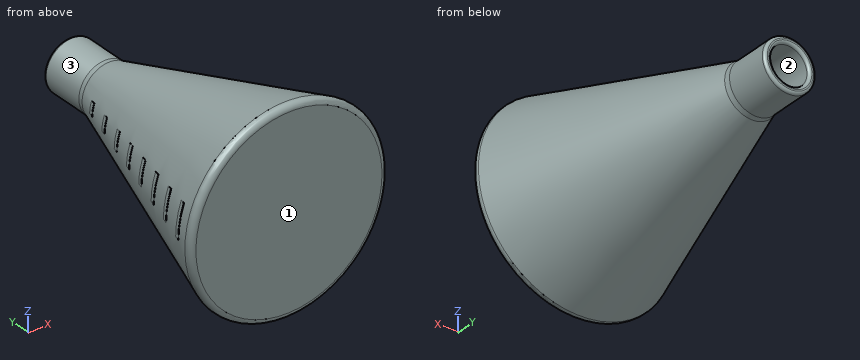
from build123d import *

# Parameters (mm, degrees)
FILLET1_R      = 7.62
FILLET2_R      = 1.27
FILLET3_R      = 2.54
FILLET4_R      = 2.54
REVOLVE2_ANGLE = 20


with BuildPart() as part:
    # Sketch2 → Revolve1 (revolve)
    with BuildSketch(Plane.XY, mode=Mode.PRIVATE) as revolve1_sk:
        Polygon((-11.704475972, 127), (-8.529475972, 127), (-8.529475972, 105.527709861), (-41.475985329, 3.175), (0, 3.175), (0, 0), (-45.672992146, 0), (-11.704475972, 105.527709861), align=None)
    revolve(revolve1_sk.sketch.rotate(Axis((0, 0, 0), (0, 1, 0)), 270), axis=Axis((0, 0, 0), (0, 1, 0)))

    # Fillet1
    fillet1_edges = [part.edges().sort_by_distance(p)[0] for p in [
        (0, 105.527709861, 11.704475972),
    ]]
    fillet(fillet1_edges, radius=FILLET1_R)

    # Fillet2
    fillet2_edges = [part.edges().sort_by_distance(p)[0] for p in [
        (0, 127, 11.704475972),
        (0, 127, 8.529475972),
    ]]
    fillet(fillet2_edges, radius=FILLET2_R)

    # Fillet3
    fillet3_edges = [part.edges().sort_by_distance(p)[0] for p in [
        (0, 0, 45.672992146),
    ]]
    fillet(fillet3_edges, radius=FILLET3_R)

    # Fillet4
    fillet4_edges = [part.edges().sort_by_distance(p)[0] for p in [
        (0, 3.175, 41.475985329),
    ]]
    fillet(fillet4_edges, radius=FILLET4_R)

    # Sketch3 → Revolve2 (revolve)
    with BuildSketch(Plane.XY):
        Polygon((-42.578605395, 9.61312368), (-42.691844754, 9.649574513), (-41.913566134, 12.067400477), (-41.800326776, 12.030949643), align=None)
        Polygon((-38.687212298, 21.702253498), (-38.800451656, 21.738704331), (-38.022173037, 24.156530295), (-37.908933678, 24.120079461), align=None)
        Polygon((-34.7958192, 33.791383316), (-34.909058559, 33.82783415), (-34.130779939, 36.245660113), (-34.017540581, 36.20920928), align=None)
        Polygon((-30.904426103, 45.880513134), (-31.017665461, 45.916963968), (-30.239386842, 48.334789931), (-30.126147483, 48.298339098), align=None)
        Polygon((-27.013033005, 57.969642952), (-27.126272364, 58.006093786), (-26.347993744, 60.42391975), (-26.234754386, 60.387468916), align=None)
        Polygon((-23.121639908, 70.058772771), (-23.234879266, 70.095223604), (-22.456600647, 72.513049568), (-22.343361288, 72.476598734), align=None)
        Polygon((-19.23024681, 82.147902589), (-19.343486169, 82.184353422), (-18.565207549, 84.602179386), (-18.451968191, 84.565728552), align=None)
        Polygon((-15.338853713, 94.237032407), (-15.452093071, 94.27348324), (-14.673814452, 96.691309204), (-14.560575093, 96.654858371), align=None)
    revolve(axis=Axis((0, 0, 0), (0, 1, 0)), revolution_arc=REVOLVE2_ANGLE)


solid = part.part
Design review of the part built by this model. Coordinates are the model's own, in mm. Face numbers are marked on the shaded views. Round coordinates to 2 decimals unless told otherwise and drop trailing zeros. Loops run counter-clockwise (first coordinate to the right, second up) from the corner with the lowest first, then second, coordinate; pieces in that order, holes last. Notation, with made-up numbers: (51.25, -17.5) - (98.25, -17.5) arc R13 ccw to (98.25, -4.5) - close; hole circle Ø7 at (56, 20.5). An arc over 180 degrees is marked (long way). One line per item, written item: value. Start each with the question number.
1) Consider section B-B on y = 27. Give the boundary of the cut face in (x, z).
2) To check wall thickness, follow L1, parallel to X at y = 112, z = 0; L2, parallel to Y at x = 6, z = 1 (3 decimals); L3, parallel to Z at x = -10, y = 80. State the ranges of each line that lie inside material, in increasing order. Write a range as from..to.
3) Insertion check: pin 1 Ø4 at (y, z) = (29.5, 4) entering from -X; pin 2 Ø5 at (x, y) = (7.5, 62) entering from -Z; pin 3 Ø10 at (x, y) = (-0.5, 84.5) entering from +Z; pin 4 Ø13.5 at (x, z) = (0, 0) entering from -Y. Each pin has a flat end and moves straight along its axis. Give the tip position at first contact, or say it passes through.
4) Draft analysis for pull direction Z (two halves, no side actions). For the marked faces 1, 2 and 3, state which applies: +Z half, -Z half, draft (parallel to the pull), parting line (faces both ways), or undercut.
5) Consider section A-A on y = 91. Give the boundary of the cut face in (x, z), then the cut area to 3 significant figures.
Reported:
1. outline: circle Ø73.96 at (0, 0); hole circle Ø67.61 at (0, 0)
2. L1: x = -11.7..-8.53, 8.53..11.7
2. L2: y = 0..3.175
2. L3: z = -17.23..-13.43, 13.43..17.23
3. pin 1: stops at x = -36.63
3. pin 2: stops at z = -25.67
3. pin 3: stops at z = 20.08
3. pin 4: stops at y = 0
4. face 1: draft
4. face 2: undercut
4. face 3: parting line
5. outline: circle Ø32.76 at (0, 0); hole circle Ø26.41 at (0, 0)
5. area: 295 mm^2
